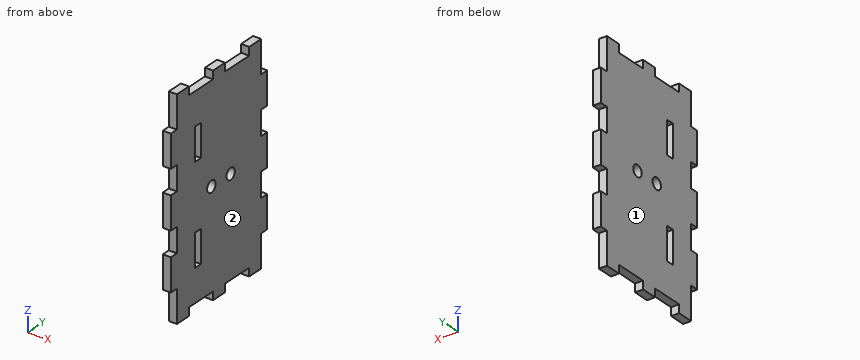
```python
from build123d import *

# Parameters (mm, degrees)
BOSS_EXTRUDE1_DEPTH = 5
SKETCH3_W           = 20
SKETCH3_H           = 5
CUT_EXTRUDE2_DEPTH  = 5
SKETCH2_R           = 3.5
CUT_EXTRUDE3_DEPTH  = 5


with BuildPart() as part:
    # Sketch1 → Boss-Extrude1 (new body)
    with BuildSketch(Plane(origin=(0, 0, 0), x_dir=(0, 0, -1), z_dir=(1, 0, 0))):
        Polygon((65, 35), (65, 25), (60, 25), (60, 5), (65, 5), (65, -5), (60, -5), (60, -25), (65, -25), (65, -35), (60, -35), (45, -35), (45, -40), (25, -40), (25, -35), (10, -35), (10, -40), (-10, -40), (-10, -35), (-25, -35), (-25, -40), (-45, -40), (-45, -35), (-60, -35), (-65, -35), (-65, -25), (-60, -25), (-60, -5), (-65, -5), (-65, 5), (-60, 5), (-60, 25), (-65, 25), (-65, 35), (-60, 35), (-45, 35), (-45, 40), (-25, 40), (-25, 35), (-10, 35), (-10, 40), (10, 40), (10, 35), (25, 35), (25, 40), (45, 40), (45, 35), (60, 35), align=None)
    extrude(amount=BOSS_EXTRUDE1_DEPTH)

    # Sketch3 → Cut-Extrude2 (cut)
    with BuildSketch(Plane(origin=(5, 0, 0), x_dir=(0, 0, -1), z_dir=(1, 0, 0))):
        with Locations((30, -17.5)):
            Rectangle(SKETCH3_W, SKETCH3_H)
        with Locations((-30, -17.5)):
            Rectangle(SKETCH3_W, SKETCH3_H)
    extrude(amount=-CUT_EXTRUDE2_DEPTH, mode=Mode.SUBTRACT)

    # Sketch2 → Cut-Extrude3 (cut)
    with BuildSketch(Plane(origin=(0, 0, 0), x_dir=(0, 0, -1), z_dir=(1, 0, 0))):
        with Locations((0, 9.623429696)):
            Circle(SKETCH2_R)
        with Locations(Location((0, -6.376570304, 0), (0, 0, 180))):
            Circle(SKETCH2_R)
    extrude(amount=CUT_EXTRUDE3_DEPTH, mode=Mode.SUBTRACT)


solid = part.part
```
Geometry check sheet. Reference: the model listing, model coordinates, mm. Face numbers are marked on the shaded views. Coordinates: 2 decimals unless noted, no trailing zeros. Order: outer loops, then holes, each group sorted by start corner. A loop starts at its lowest first (then second) coordinate and runs counter-clockwise, first axis right, second up. Notation, with made-up numbers: (84, 23) - (129, 23) arc R33 ccw to (129, 60) - close; hole circle Ø8 at (53.25, 69.5). An arc over 180 degrees is marked (long way). Answer as a JSON object with one key per item and string values. Group by question number.
Item 1: Draft check along X on the marked faces 1 and 2. Enter one of: +X half, -X half, draft (parallel to the pull), parting line (faces both ways), or undercut.
Item 2: Scan lines: probe 1 along Y at (x, z) = (1.3, 0); probe 2 along Y at (x, z) = (0.25, -38); probe 3 along Y at (x, z) = (1.85, 1.5). Record each from-to range of solid material in increasing order.
Item 3: Sectioned sample at B-B, the plane z = 0. Record the cut outline in (x, y), and give its area (3 significant figures).
Item 4: Sectioned sample at A-A, the plane z = 32. Record the cut outline in (x, y).
Item 5: Sectioned sample at C-C, the plane x = 2.45. Give the number of separate pieces and of enclosed holes in the cut face, and give its area (3 significant figures).
Item 6: Depth check by flat-ended pin: pin 1 Ø1.5 at (x, y) = (3, 36.5) entering from +Z; pin 2 Ø1 at (x, z) = (4.5, 50) entering from -Y; pin 3 Ø1.5 at (x, y) = (3, 37.5) entering from -Z. Enter the tip coordinate at first touch or a pass-through.
Resolved:
{
 "1": {"face 1": "-X half", "face 2": "+X half"},
 "2": {"probe 1": "-40 to -9.88, -2.88 to 6.12, 13.12 to 40", "probe 2": "-40 to -20, -15 to 40", "probe 3": "-40 to -9.54, -3.21 to 6.46, 12.79 to 40"},
 "3": {"outline": "(0, -40) - (5, -40) - (5, -9.88) - (0, -9.88) - close; (0, -2.88) - (5, -2.88) - (5, 6.12) - (0, 6.12) - close; (0, 13.12) - (5, 13.12) - (5, 40) - (0, 40) - close", "area": "330 mm^2"},
 "4": {"outline": "(0, -40) - (5, -40) - (5, -20) - (0, -20) - close; (0, -15) - (5, -15) - (5, 40) - (0, 40) - close"},
 "5": {"separate pieces": "1", "enclosed holes": "4", "area": "9,020 mm^2"},
 "6": {"pin 1": "z = 45", "pin 2": "y = -35", "pin 3": "z = -45"}
}
